```python
from build123d import *

# Parameters (mm, degrees)
SKETCH1_R           = 1.25
BOSS_EXTRUDE1_DEPTH = 10
SKETCH2_W           = 10.5
SKETCH2_H           = 5.5
CUT_EXTRUDE1_DEPTH  = 55


with BuildPart() as part:
    # Sketch1 → Boss-Extrude1 (new body)
    with BuildSketch(Plane(origin=(0, 0, 0), x_dir=(1, 0, 0), z_dir=(0, 1, 0))):
        Polygon((10, -5), (22.5, -5), (22.5, 5), (2.5, 5), (2.5, -15), (-2.5, -15), (-2.5, 5), (-22.5, 5), (-22.5, -5), (-10, -5), (-10, -70), (10, -70), align=None)
        with Locations(Location((-15.875, 0, 0), (0, 0, 270))):
            Circle(SKETCH1_R, mode=Mode.SUBTRACT)
        with Locations(Location((15.875, 0, 0), (0, 0, 270))):
            Circle(SKETCH1_R, mode=Mode.SUBTRACT)
    extrude(amount=BOSS_EXTRUDE1_DEPTH)

    # Sketch2 → Cut-Extrude1 (cut)
    with BuildSketch(Plane.XY.offset(70)):
        with Locations((0, 5)):
            Rectangle(SKETCH2_W, SKETCH2_H)
    extrude(amount=-CUT_EXTRUDE1_DEPTH, mode=Mode.SUBTRACT)


solid = part.part
```
Source: CAD feature listing. Evaluate the final solid. Frame: model axes, mm. A direction names the side the tool comes from. Give positions to 0.01 mm unless a question says otherwise; leave off trailing zeros. Order: outer loops, then holes, each group sorted by start corner. A loop starts at its lowest first (then second) coordinate and runs counter-clockwise, first axis right, second up. Notation, with made-up numbers: (79.25, 71) -> (87.25, 71) arc R4 ccw to (87.25, 75) -> close; hole circle Ø4 at (-21, 55). An arc over 180 degrees is marked (long way). Use a Markdown table: item, result.
Q1. Section A-A (z = 0). Return the cut outline in (x, y) (3 decimals).
A:
| item | result |
|---|---|
| outline | (-22.5, 0) -> (-17.125, 0) -> (-17.125, 10) -> (-22.5, 10) -> close; (-14.625, 0) -> (-2.5, 0) -> (-2.5, 10) -> (-14.625, 10) -> close; (2.5, 0) -> (14.625, 0) -> (14.625, 10) -> (2.5, 10) -> close; (17.125, 0) -> (22.5, 0) -> (22.5, 10) -> (17.125, 10) -> close |
Q2. Section C-C (z = 43.5). Return the cut outline in (x, y), and give its area (3 significant figures).
A:
| item | result |
|---|---|
| outline | (-10, 0) -> (10, 0) -> (10, 10) -> (-10, 10) -> close; hole (-5.25, 2.25) -> (5.25, 2.25) -> (5.25, 7.75) -> (-5.25, 7.75) -> close |
| area | 142 mm^2 |
Q3. First-contact query: P1, Ø2, axis at y = 2, z = 9.5, coming from the +X side; P2, Ø6, axis at y = 4, z = 39, coming from the -X side; P3, Ø0.8, axis at x = 4, y = 4.5, coming from the +Z side; P4, Ø2, axis at x = -15.875, z = 0, coming from the +Y side. Flat tips, straight axial feed; report the tip coordinate or a pass-through.
A:
| item | result |
|---|---|
| P1 | x = 10 |
| P2 | x = -10 |
| P3 | z = 15 |
| P4 | through |
Q4. Pull-direction query (X, two-part tool) for faces 1 (the face through (10, 5, 38)), 2 (the face through (-14.636, 4.93, -0.163)), 3 (the face through (16.93, 4.93, 0.67)), 4 (the face through (16, 5, 5)); classes: +X half, -X half, draft (parallel to the pull), parting line (faces both ways), or undercut.
A:
| item | result |
|---|---|
| face 1 | +X half |
| face 2 | undercut |
| face 3 | undercut |
| face 4 | draft |
Q5. Section D-D (y = 1). Return the cut outline in (x, z) (3 decimals), and give its area (3 significant figures).
A:
| item | result |
|---|---|
| outline | (-22.5, -5) -> (-2.5, -5) -> (-2.5, 15) -> (2.5, 15) -> (2.5, -5) -> (22.5, -5) -> (22.5, 5) -> (10, 5) -> (10, 70) -> (-10, 70) -> (-10, 5) -> (-22.5, 5) -> close; hole circle Ø2.5 at (-15.875, 0); hole circle Ø2.5 at (15.875, 0) |
| area | 1,640 mm^2 |
Q6. Material intervals for line 1 (X direction, y = 3.25, z = 0) (3 decimals); line 2 (Y direction, x = -4, z = 47); line 3 (X direction, y = 4, z = 8), sorted ascending. Write a range as [from, to].
A:
| item | result |
|---|---|
| line 1 | [-22.5, -17.125], [-14.625, -2.5], [2.5, 14.625], [17.125, 22.5] |
| line 2 | [0, 2.25], [7.75, 10] |
| line 3 | [-10, -2.5], [2.5, 10] |
Q7. Section B-B (y = 6.5). Return the cut outline in (x, z) (3 decimals), and give its area (3 significant figures).
A:
| item | result |
|---|---|
| outline | (-22.5, -5) -> (-2.5, -5) -> (-2.5, 15) -> (-5.25, 15) -> (-5.25, 70) -> (-10, 70) -> (-10, 5) -> (-22.5, 5) -> close; (2.5, -5) -> (22.5, -5) -> (22.5, 5) -> (10, 5) -> (10, 70) -> (5.25, 70) -> (5.25, 15) -> (2.5, 15) -> close; hole circle Ø2.5 at (-15.875, 0); hole circle Ø2.5 at (15.875, 0) |
| area | 1,060 mm^2 |
Q8. Access query for faces 5 (the face through (-16, 5, 5)), 6 (the face through (0, 9, 15)), 7 (the face through (5.25, 5, 43)). Directions: +Z, -Z, +X, -X, +Y, -Y. A direction counts if a zero-diameter tool reaches every point of the face in a straight line with its end or side. Return the directions, or none.
A:
| item | result |
|---|---|
| face 5 | +Z, -X, +Y, -Y |
| face 6 | -Z, +Y, -Y |
| face 7 | +Z |
